Could you check a few things on this drawing? It's one solid part, dimensions in mm from its lowest x, y, z. A direction names the side the tool comes from. Round coordinates to 2 decimals unless told otherwise and drop trailing zeros. Write each loop counter-clockwise with the first axis right and the second up, starting at its lowest first coordinate (ties: lowest second). Pieces come first, ordered by that corner, then holes. Notation, with made-up numbers: (54.25, -31) -> (68.25, -31) arc R19 cw to (68.25, -14) -> close; hole circle Ø3 at (70, 63.25). An arc over 180 degrees is marked (long way). Return JSON: item names as keys, results as strings.
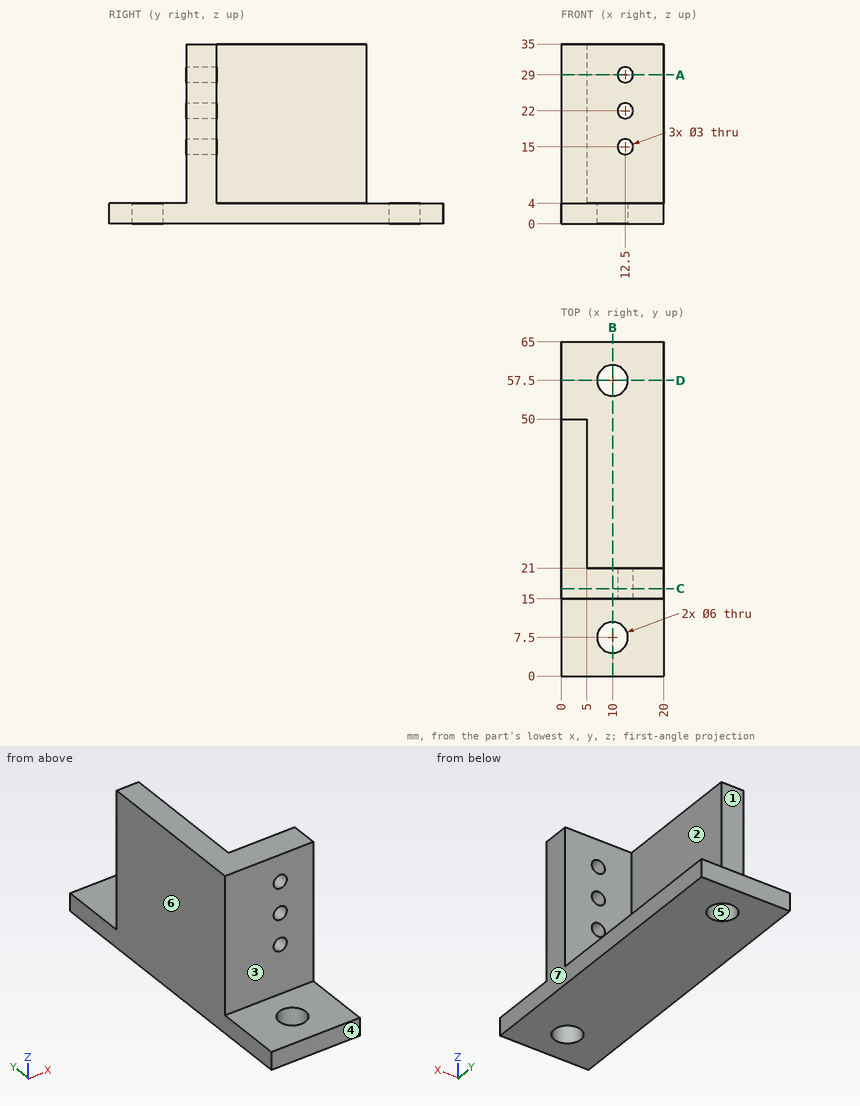
1) Will these pins go through, and if not, where does the flat tip stop? pin 1 Ø4 at (x, z) = (12.5, 29) entering from +Y; pin 2 Ø10 at (x, z) = (10, 27.5) entering from -Y; pin 3 Ø8 at (x, y) = (4.5, 8) entering from +Z.
Return value:
{"pin 1": "y = 21", "pin 2": "y = 15", "pin 3": "z = 4"}
2) I want a section at C-C, the plane y = 17. Please give me the cut outline in (x, z), and give its area (3 significant figures).
Return value:
{"outline": "(0, 0) -> (20, 0) -> (20, 35) -> (0, 35) -> close; hole circle Ø3 at (12.5, 15); hole circle Ø3 at (12.5, 22); hole circle Ø3 at (12.5, 29)", "area": "679 mm²"}
3) Thinking about a two-plate mould opening in X: for the marked faces 4, 5, 6 and 7, which applies, pulls with the +X half, pulls with the -X half, needs draft (parallel to the pull), parting line crosses it, or undercut?
Return value:
{"face 4": "needs draft", "face 5": "undercut", "face 6": "pulls with the -X half", "face 7": "pulls with the +X half"}
4) For the marked faces 1, 2 and 3, which set-ups out of +Z, -Z, +X, -X, +Y, -Y let a thin tool reach every point of the face, with its end or its side?
Return value:
{"face 1": "+Z, +X, -X, +Y", "face 2": "+Z, +X, +Y", "face 3": "+Z, +X, -X, -Y"}
5) I want a section at D-D, the plane y = 57.5. Please give me the cut outline in (x, z).
Return value:
{"outline": "(0, 0) -> (7, 0) -> (7, 4) -> (0, 4) -> close; (13, 0) -> (20, 0) -> (20, 4) -> (13, 4) -> close"}
6) I want a section at A-A, the plane z = 29. Please give me the cut outline in (x, y).
Return value:
{"outline": "(0, 15) -> (11, 15) -> (11, 21) -> (5, 21) -> (5, 50) -> (0, 50) -> close; (14, 15) -> (20, 15) -> (20, 21) -> (14, 21) -> close"}
7) If I drill on probe 1 along Z at (x, y) = (12.5, 16.2); probe 2 along Y at (x, z) = (15, 31); probe 3 along Z at (x, y) = (18, 52), over which ranges is the centre line in solid material (lowest first)? Write a range as [from, to].
Return value:
{"probe 1": "[0, 13.5], [16.5, 20.5], [23.5, 27.5], [30.5, 35]", "probe 2": "[15, 21]", "probe 3": "[0, 4]"}
8) I want a section at B-B, the plane x = 10. Please give me the cut outline in (y, z), and give its area (3 significant figures).
Return value:
{"outline": "(0, 0) -> (4.5, 0) -> (4.5, 4) -> (0, 4) -> close; (10.5, 0) -> (54.5, 0) -> (54.5, 4) -> (21, 4) -> (21, 35) -> (15, 35) -> (15, 4) -> (10.5, 4) -> close; (60.5, 0) -> (65, 0) -> (65, 4) -> (60.5, 4) -> close", "area": "398 mm²"}
